from build123d import *

# Parameters (mm, degrees)
SKETCH1_R           = 11.4
BOSS_EXTRUDE1_DEPTH = 8
SKETCH2_OUTSIDE_W   = 38.236
SKETCH2_OUTSIDE_H   = 38.236
SKETCH2_OUTSIDE_R   = 9
CUT_EXTRUDE1_DEPTH  = 8
CUT_EXTRUDE1_DRAFT  = -23
SKETCH3_R           = 1.1
CUT_EXTRUDE2_DEPTH  = 8
CUT_EXTRUDE3_DEPTH  = 6
CIRPATTERN1_COUNT   = 2
SKETCH5_R           = 7.75
CUT_EXTRUDE5_DEPTH  = 6.5


with BuildPart() as part:
    # Sketch1 → Boss-Extrude1 (new body)
    with BuildSketch(Plane(origin=(0, 0, 0), x_dir=(1, 0, 0), z_dir=(0, 1, 0))):
        with Locations(Location((0, 0, 0), (0, 0, 270))):
            Circle(SKETCH1_R)
    extrude(amount=BOSS_EXTRUDE1_DEPTH)


with BuildPart() as cut_extrude1_tool:
    # Sketch2 outside → Cut-Extrude1 (with draft: the straight prism first)
    with BuildSketch(Plane(origin=(0, 8, 0), x_dir=(1, 0, 0), z_dir=(0, 1, 0))):
        Rectangle(SKETCH2_OUTSIDE_W, SKETCH2_OUTSIDE_H)
        Circle(SKETCH2_OUTSIDE_R, mode=Mode.SUBTRACT)
    extrude(amount=-CUT_EXTRUDE1_DEPTH)
    # Cut-Extrude1: the draft: its side faces are tilted about the plane it starts from
    cut_extrude1_sides = [cut_extrude1_tool.faces().sort_by_distance(p)[0] for p in [
        (0, 4, 19.118),
        (19.118, 4, 0),
        (0, 4, -19.118),
        (-19.118, 4, 0),
        (-9, 4, 0),
    ]]
    draft(cut_extrude1_sides, Plane(origin=(0, 8, 0), x_dir=(1, 0, 0), z_dir=(0, 1, 0)), CUT_EXTRUDE1_DRAFT)


with BuildPart() as part_1:
    add(part.part)

    # Cut-Extrude1: cut by cut_extrude1_tool
    add(cut_extrude1_tool.part, mode=Mode.SUBTRACT)

    # Sketch3 → Cut-Extrude2 (cut)
    with BuildSketch(Plane.XZ):
        with Locations(Location((-6.610810867, 7.503144653, 0), (0, 0, 270))):
            Circle(SKETCH3_R)
    cut_extrude2 = extrude(amount=-CUT_EXTRUDE2_DEPTH, mode=Mode.SUBTRACT)

    # Sketch4 → Cut-Extrude3 (cut)
    with BuildSketch(Plane(origin=(0, 8, 0), x_dir=(1, 0, 0), z_dir=(0, 1, 0))):
        with BuildLine():
            Line((-8.111439797, -6.18098248), (-10.53240187, -8.928728406))
            Line((-10.53240187, -8.928728406), (-7.531144009, -11.573052753))
            Line((-7.531144009, -11.573052753), (-5.110181936, -8.825306826))
            ThreePointArc((-5.110181936, -8.825306826), (-5.288648693, -6.002515722), (-8.111439797, -6.18098248))
        make_face()
    cut_extrude3 = extrude(amount=-CUT_EXTRUDE3_DEPTH, mode=Mode.SUBTRACT)

    # CirPattern1: Cut-Extrude2, Cut-Extrude3 ×2 about axis
    cirpattern1_axis = Axis((0, 0, 0), (0, 1, 0))
    add([cut_extrude2.rotate(cirpattern1_axis, i * 360 / CIRPATTERN1_COUNT) for i in range(1, CIRPATTERN1_COUNT)], mode=Mode.SUBTRACT)
    add([cut_extrude3.rotate(cirpattern1_axis, i * 360 / CIRPATTERN1_COUNT) for i in range(1, CIRPATTERN1_COUNT)], mode=Mode.SUBTRACT)

    # Sketch5 → Cut-Extrude5 (cut)
    with BuildSketch(Plane.XZ):
        with Locations(Location((0, 0, 0), (0, 0, 270))):
            Circle(SKETCH5_R)
    extrude(amount=-CUT_EXTRUDE5_DEPTH, mode=Mode.SUBTRACT)


solid = part_1.part
Source: CAD feature listing. Evaluate the final solid. Frame: model axes, mm. A direction names the side the tool comes from. Round coordinates to 2 decimals unless told otherwise and drop trailing zeros. Order: outer loops, then holes, each group sorted by start corner. A loop starts at its lowest first (then second) coordinate and runs counter-clockwise, first axis right, second up. Notation, with made-up numbers: (-17.5, 89) - (41.5, 89) arc R35 cw to (41.5, 127) - close; hole circle Ø1 at (-1, 19). An arc over 180 degrees is marked (long way). Use a Markdown table: item, result. Add a question column.
1. Set-up query: faces 4 (the flat face through (8.42, 3.26, -6.53)), 5 (the flat face through (0, 6.5, 0)), 6 (the flat face through (5.43, 3.26, -9.19)), 7 (the flat face through (-8.42, 3.26, 6.53)). Return all of +Z, -Z, +X, -X, +Y, -Y with unobstructed straight access to the full face (end or side cutting, diameter ignored); none if empty.
2. Section query A-A (z = 0). Return the cut outline in (x, y), then the cut area to 3 significant figures.
3. Section query C-C (y = 4). Return the cut outline in (x, z), then the cut area to 3 significant figures.
4. Line query: probe 1 along Y at (x, z) = (1.5, 5); probe 2 along Z at (x, y) = (2.75, 2); probe 3 along Z at (x, y) = (6.5, 1.5). Output: solid intervals per line, ascending.
5. Section query D-D (y = 7). Return the cut outline in (x, z), then the cut area to 3 significant figures.
6. Mould query, pull axis Z, two halves, no side actions, for faces 1 (the flat face through (0, 8, 0)), 2 (the conical face through (7.115, 6.469, 6.519)), 3 (the flat face through (-5, 2, 7)). Classes: +Z half, -Z half, draft (parallel to the pull), parting line (faces both ways), or undercut.
7. First-contact query: pin 1 (1.5 mm diameter, centred on y = 5, z = 5.5, fed in from -X); pin 2 (2.5 mm diameter, centred on x = -6.61, z = 7.5, fed in from +Y); pin 3 (3 mm diameter, centred on y = 6, z = -4, fed in from -X). Flat tips, straight axial feed; report the tip coordinate or a pass-through.
8. Section query B-B (x = 0). Return the cut outline in (y, z), then the cut area to 3 significant figures.
Derived:
| question | item | result |
|---|---|---|
| 1 | face 4 | -Z, +Y |
| 1 | face 5 | -Y |
| 1 | face 6 | +X, +Y |
| 1 | face 7 | +Z, +Y |
| 2 | outline | (-11.4, 0) - (-7.75, 0) - (-7.75, 6.5) - (7.75, 6.5) - (7.75, 0) - (11.4, 0) - (11.4, 2.35) - (9, 8) - (-9, 8) - (-11.4, 2.35) - close |
| 2 | area | 68.1 mm2 |
| 3 | outline | (-8.45, 6.56) arc R10.7 ccw to (5.45, -9.21) - (5.11, -8.83) arc R2 cw to (8.11, -6.18) - (8.45, -6.56) arc R10.7 ccw to (-5.45, 9.21) - (-5.11, 8.83) arc R2 cw to (-8.11, 6.18) - close; hole circle Ø15.5 at (0, 0) |
| 3 | area | 153 mm2 |
| 4 | probe 1 | 6.5 to 8 |
| 4 | probe 2 | -11.06 to -7.25, 7.25 to 11.06 |
| 4 | probe 3 | -9.37 to -8.6, -6.41 to -4.22, 4.22 to 9.37 |
| 5 | outline | (-7.5, 5.71) arc R9.42 ccw to (4.72, -8.16) arc R2 cw to (7.5, -5.71) arc R9.42 ccw to (-4.72, 8.16) arc R2 cw to start |
| 5 | area | 271 mm2 |
| 6 | face 1 | draft |
| 6 | face 2 | parting line |
| 6 | face 3 | undercut |
| 7 | pin 1 | x = -9.25 |
| 7 | pin 2 | y = 2 |
| 7 | pin 3 | x = -9.88 |
| 8 | outline | (0, -11.4) - (2.35, -11.4) - (8, -9) - (8, 9) - (2.35, 11.4) - (0, 11.4) - (0, 7.75) - (6.5, 7.75) - (6.5, -7.75) - (0, -7.75) - close |
| 8 | area | 68.1 mm2 |
